Input: part model. Units: mm. Frame: model coordinates. A direction names the side the tool comes from. Give positions to 0.01 mm unless a question says otherwise; leave off trailing zeros. Loops run counter-clockwise (first coordinate to the right, second up) from the corner with the lowest first, then second, coordinate; pieces in that order, holes last. Notation, with made-up numbers: (6, 70.25) - (17, 70.25) arc R23 ccw to (17, 91.25) - close; hole circle Ø9 at (39.25, 51). An arc over 180 degrees is marked (long way). Answer as a JSON object with one key per item and string values. Group by question number.
(1) Section query A-A (z = -4.5). Return loops of the section in (x, y), plus the area to 3 significant figures.
(2) Access query for faces 5 (the conical face through (0.93, 4.187, 1.397)), 6 (the cylindrical face through (0.585, 2.636, -3.143)). Directions: +Z, -Z, +X, -X, +Y, -Y. A direction counts if a zero-diameter tool reaches every point of the face in a straight line with its end or side. Return the directions, or none.
(3) Mould query, pull axis Z, two halves, no side actions, for faces 1 (the flat face through (0, 0, 12.86)), 2 (the flat face through (-3, 0, 0)), 3 (the conical face through (0.524, 2.362, 4.925)), 4 (the cylindrical face through (-3.35, 6.43, 0.49)). Classes: +Z half, -Z half, draft (parallel to the pull), parting line (faces both ways), or undercut.
(4) Section query B-B (z = 6). Return loops of the section in (x, y), plus the area to 3 significant figures.
(5) Pin query (flat end, axial travel): P1, Ø1.5, axis at y = -3, z = -4, coming from the -X side; P2, Ø8, axis at y = -4.5, z = 2, coming from the -X side; P3, Ø6, axis at y = -2, z = 5, coming from the +X side. Return the tip coordinate at first contact, or that it passes through.
(6) Material intervals for L1, parallel to X at y = 1.5, z = 12.25; L2, parallel to Z at x = 3.5, y = -0.25; L3, parallel to Y at x = 0.5, z = 9, sorted ascending.
```python
from build123d import *


with BuildPart() as f1:
    # F0 (on Front) → F1 (revolve)
    with BuildSketch(Plane.XZ):
        with BuildLine():
            Line((-2.7, -6.2), (0, -6.2))
            Line((0, -6.2), (0, 12.86))
            Line((0, 12.86), (-2.630608, 12.86))
            ThreePointArc((-2.630608, 12.86), (-3.975502, 10.199833), (-3.101612, 7.35))
            Line((-3.101612, 7.35), (-2.950293, 7.35))
            ThreePointArc((-2.950293, 7.35), (-2.338286, 7.065216), (-2.162004, 6.413618))
            Line((-2.162004, 6.413618), (-2.812344, 2.65465))
            ThreePointArc((-2.812344, 2.65465), (-3.250065, 1.829751), (-4.090995, 1.423678))
            Line((-4.090995, 1.423678), (-7.25, 1))
            Line((-7.25, 1), (-7.25, 0))
            Line((-7.25, 0), (-2.7, 0))
            Line((-2.7, 0), (-2.7, -6.2))
        make_face()
    revolve(axis=Axis((0, 0, 1.878261), (0, 0, 1)))


solid = f1.part
```
Recorded:
{
 "1": {"outline": "circle Ø5.4 at (0, 0)", "area": "22.9 mm^2"},
 "2": {"face 5": "+Z", "face 6": "-Z"},
 "3": {"face 1": "+Z half", "face 2": "-Z half", "face 3": "undercut", "face 4": "draft"},
 "4": {"outline": "circle Ø4.47 at (0, 0)", "area": "15.7 mm^2"},
 "5": {"P1": "stops at x = -1.49", "P2": "stops at x = -7.22", "P3": "stops at x = 3.29"},
 "6": {"L1": "x = -2.82 to 2.82", "L2": "z = 0 to 1.63, 7.96 to 11.76", "L3": "y = -3.86 to 3.86"}
}
